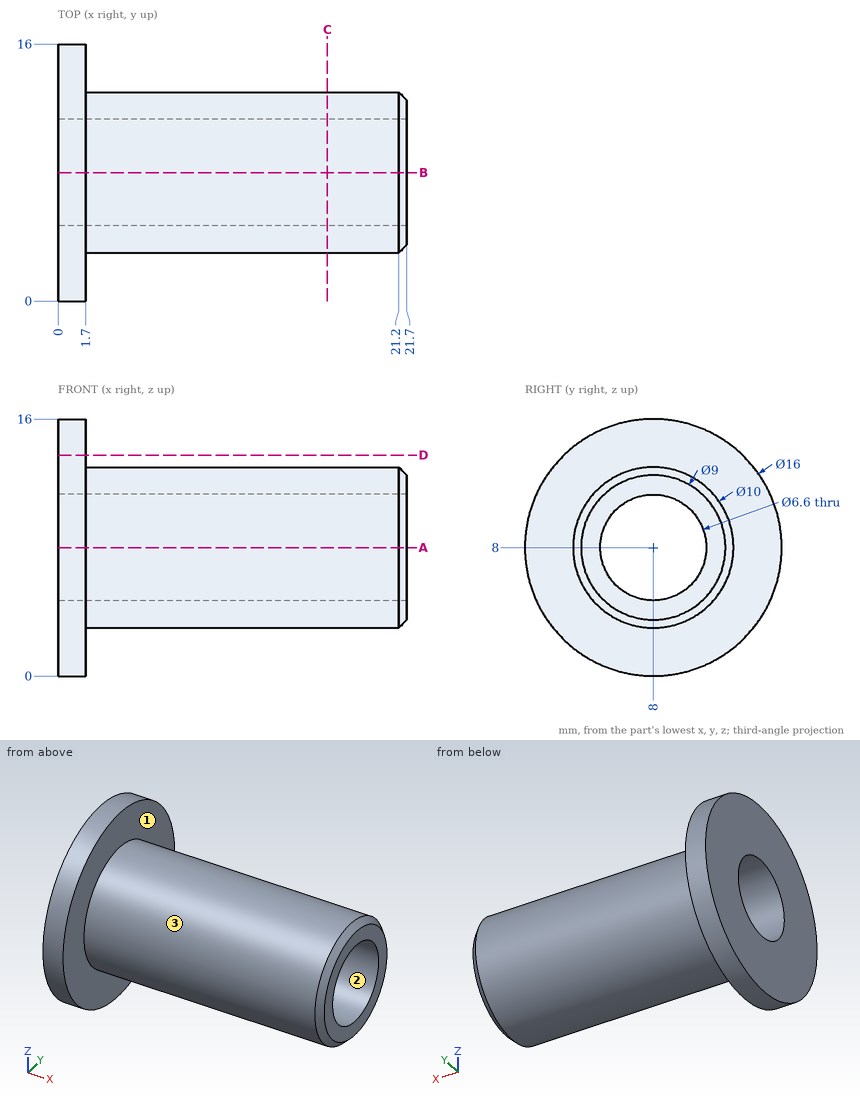
Can you work these out from the drawing? Everything is in mm from the part's minimum corner. Give positions to 0.01 mm unless a question says otherwise; leave off trailing zeros. Loops run counter-clockwise (first coordinate to the right, second up) from the corner with the lowest first, then second, coordinate; pieces in that order, holes last. Notation, with made-up numbers: (14, -16.5) -> (25, -16.5) arc R19 cw to (25, 18.5) -> close; hole circle Ø8 at (5.5, 49.25). An arc over 180 degrees is marked (long way). Write item = value, one per line.
1) Suppose I cut it at D-D on z = 13.75. Write out the boundary of the cut face in (x, y).
Check result:
outline = (0, 2.44) -> (1.7, 2.44) -> (1.7, 13.56) -> (0, 13.56) -> close
2) Thinking about a two-plate mould opening in Z: for the marked faces 1, 2 and 3, which applies, released by +Z, released by -Z, zero draft, split by the parting line, or undercut?
Check result:
face_1 = zero draft
face_2 = undercut
face_3 = split by the parting line
3) Will these pins go through, and if not, where does the flat tip stop? pin 1 (8 mm diameter, centred on x = 4.5, z = 8, fed in from +Y); pin 2 (1 mm diameter, centred on x = 4.5, y = 13, fed in from +Z); pin 3 (2 mm diameter, centred on x = 12.5, z = 9.5, fed in from -Y); pin 4 (1.5 mm diameter, centred on x = 13.5, y = 9.5, fed in from -Z).
Check result:
pin_1 = 16
pin_2 = 10.18
pin_3 = 3.03
pin_4 = 3.06
4) Suppose I cut it at A-A on z = 8. Write out the boundary of the cut face in (x, y).
Check result:
outline = (0, 0) -> (1.7, 0) -> (1.7, 3) -> (21.2, 3) -> (21.7, 3.5) -> (21.7, 4.7) -> (0, 4.7) -> close; (0, 11.3) -> (21.7, 11.3) -> (21.7, 12.5) -> (21.2, 13) -> (1.7, 13) -> (1.7, 16) -> (0, 16) -> close
5) Suppose I cut it at C-C on x = 16.75. Write out the boundary of the cut face in (y, z).
Check result:
outline = circle Ø10 at (8, 8); hole circle Ø6.6 at (8, 8)
6) I need wall thicknesses on L1, parallel to Z at x = 13.75, y = 8; L2, parallel to X at y = 1, z = 11; L3, parallel to Y at x = 12.25, z = 10.5. Which ranges of each line are inside material? Lowest first, please. Write a range as from..to.
Check result:
L1 = 3..4.7, 11.3..13
L2 = 0..1.7
L3 = 3.67..5.85, 10.15..12.33
